Geometry: final body of the model. Coordinates: model frame, mm. A direction names the side the tool comes from. Coordinates: 2 decimals unless noted, no trailing zeros. Order: outer loops, then holes, each group sorted by start corner. A loop starts at its lowest first (then second) coordinate and runs counter-clockwise, first axis right, second up. Notation, with made-up numbers: (8.5, 42) -> (43.5, 42) arc R14 ccw to (43.5, 67) -> close; hole circle Ø10 at (43, -21.75). An arc over 180 degrees is marked (long way). Use one line per item in the form item = value.
```python
from build123d import *

# Parameters (mm, degrees)
Y_KSEKLIK_EKSTR_ZYON1_DEPTH = 40
IZIM3_R                     = 1.75
KES_EKSTR_ZYON2_DEPTH       = 3
IZIM4_R                     = 1.75
IZIM4_R_2                   = 6.898282176
KES_EKSTR_ZYON3_DEPTH       = 37


with BuildPart() as part:
    # Çizim1 → Yükseklik-Ekstrüzyon1 (new body)
    with BuildSketch(Plane(origin=(0, 0, 0), x_dir=(1, 0, 0), z_dir=(0, 1, 0))):
        Polygon((0, 0), (-35, 0), (-35, -3), (12, -40.980762114), (12, -80.980762114), (15, -80.980762114), (15, -40.980762114), (0, -15), align=None)
        Polygon((-3, -15), (-3, -3), (-31, -3), (8.501534624, -34.921242333), align=None, mode=Mode.SUBTRACT)
    extrude(amount=Y_KSEKLIK_EKSTR_ZYON1_DEPTH)

    # Çizim3 → Kes-Ekstrüzyon2 (cut)
    with BuildSketch(Plane(origin=(0, 0, 0), x_dir=(0, 0, -1), z_dir=(1, 0, 0))):
        with Locations((-7.5, 20)):
            Circle(IZIM3_R)
        with Locations((-7.5, 30)):
            Circle(IZIM3_R)
        with Locations((-7.5, 10)):
            Circle(IZIM3_R)
    extrude(amount=-KES_EKSTR_ZYON2_DEPTH, mode=Mode.SUBTRACT)

    # Çizim4 → Kes-Ekstrüzyon3 (cut)
    with BuildSketch(Plane(origin=(15, 0, 0), x_dir=(0, 0, -1), z_dir=(1, 0, 0))):
        with Locations((-60.980762114, 35.5)):
            Circle(IZIM4_R)
        with Locations((-47.557368355, 27.75)):
            Circle(IZIM4_R)
        with Locations((-47.557368355, 12.25)):
            Circle(IZIM4_R)
        with Locations((-60.980762114, 4.5)):
            Circle(IZIM4_R)
        with Locations((-74.404155872, 12.25)):
            Circle(IZIM4_R)
        with Locations((-74.404155872, 27.75)):
            Circle(IZIM4_R)
        with Locations((-64.054903201, 14.675431446)):
            Circle(IZIM4_R_2)
    extrude(amount=-KES_EKSTR_ZYON3_DEPTH, mode=Mode.SUBTRACT)


solid = part.part
```
1) Section D-D, the plane z = 7.5. Output: boundary loops of the cut face in (x, y).
Results found:
outline = (-29.43, 0) -> (-25.43, 0) -> (-25.43, 40) -> (-29.43, 40) -> close; (-3, 0) -> (0, 0) -> (0, 8.25) -> (-3, 8.25) -> close; (-3, 11.75) -> (0, 11.75) -> (0, 18.25) -> (-3, 18.25) -> close; (-3, 21.75) -> (0, 21.75) -> (0, 28.25) -> (-3, 28.25) -> close; (-3, 31.75) -> (0, 31.75) -> (0, 40) -> (-3, 40) -> close
2) Pull-direction query (X, two-part tool) for faces 4 (the flat face through (-35, 20, 1)), 5 (the cylindrical face through (13.521, 12.776, 72.735)), 6 (the flat face through (-11.526, 19.72, 18.737)); classes: released by +X, released by -X, zero draft, split by the parting line, or undercut.
Results found:
face_4 = released by -X
face_5 = zero draft
face_6 = undercut
3) Section B-B, the plane z = 25. Output: boundary loops of the cut face in (x, y).
Results found:
outline = (-7.78, 0) -> (-3.78, 0) -> (-3.78, 40) -> (-7.78, 40) -> close; (2.77, 0) -> (5.77, 0) -> (5.77, 40) -> (2.77, 40) -> close
4) Access query for faces 1 (the flat face through (-3, 20, 10)), 2 (the flat face through (12, 24, 61)), 3 (the cylindrical face through (-1.5, 11.5, 6.6)). Directions: +Z, -Z, +X, -X, +Y, -Y. A direction counts if a zero-diameter tool reaches every point of the face in a straight line with its end or side. Return the directions, or none.
Results found:
face_1 = +Y, -Y
face_2 = +Z, -X, +Y, -Y
face_3 = +X
5) Contact query for flat-ended pins moving along their axis: P1, Ø4.5, axis at y = 35.5, z = 60.98, coming from the -X side; P2, Ø10, axis at y = 28.5, z = 41, coming from the -X side; P3, Ø5.5, axis at y = 27.75, z = 47.56, coming from the +X side; P4, Ø1, axis at x = 9.5, y = 35.5, coming from the -Z side. Output: stop coordinate, or through.
Results found:
P1 = 12
P2 = 5.84
P3 = 15
P4 = 30.59
6) Material intervals for probe 1 along X at (y, z) = (19, 17); probe 2 along Z at (x, y) = (-12, 11.5); probe 3 along X at (y, z) = (31, 19), sorted ascending. Write a range as from..to.
Results found:
probe_1 = -17.68..-13.68, -1.85..1.15
probe_2 = 0..3, 18.35..21.59
probe_3 = -15.2..-11.2, -0.69..2.31
7) Section A-A, the plane y = 35.5. Output: boundary loops of the cut face in (x, z), and give its area (3 significant figures).
Results found:
outline = (-35, 0) -> (0, 0) -> (0, 15) -> (15, 40.98) -> (15, 59.23) -> (12, 59.23) -> (12, 40.98) -> (-35, 3) -> close; (12, 62.73) -> (15, 62.73) -> (15, 80.98) -> (12, 80.98) -> close; hole (-31, 3) -> (-3, 3) -> (-3, 15) -> (8.5, 34.92) -> close
area = 468 mm2
8) Section C-C, the plane x = -6. Output: boundary loops of the cut face in (y, z).
Results found:
outline = (0, 0) -> (40, 0) -> (40, 3) -> (0, 3) -> close; (0, 23.2) -> (40, 23.2) -> (40, 26.43) -> (0, 26.43) -> close
